Could you check a few things on this model? Use its own coordinates, in mm. A direction names the side the tool comes from. Give positions to 0.01 mm unless a question says otherwise; leave off trailing zeros. Loops run counter-clockwise (first coordinate to the right, second up) from the corner with the lowest first, then second, coordinate; pieces in that order, holes last. Notation, with made-up numbers: (-12, 65.25) - (45, 65.25) arc R9 ccw to (45, 77.25) - close; hole circle Ø2 at (-8.75, 67). An arc over 180 degrees is marked (long way). Answer in a Markdown table with one row per item. Add a question column.
Autodesk Inventor part; units mm, degrees
ref_plane "YZ Plane" through (0, 0, 0) normal (1, 0, 0) x (0, 1, 0)
ref_plane "XZ Plane" through (0, 0, 0) normal (0, 1, 0) x (-1, 0, 0)
ref_plane "XY Plane" through (0, 0, 0) normal (0, 0, 1) x (1, 0, 0)
sketch "Sketch1" plane through (0, 0, 0) normal (0, 0, 1) x (1, 0, 0)
  line L0 (0, 0) -> (114, 0)
  arc A0 (114, 0) -> (114, 18) centre (114, 9) ccw
  arc A1 (0, 21) -> (0, 0) centre (0, 10.5) ccw
  line L1 (0, 21) -> (20.7846, 18)
  line L2 (20.7846, 18) -> (114, 18)
  circle A2 centre (114, 9) radius 4.5
  dimension "d0" = 114
  dimension "d1" = 18
  dimension "d2" = 9
  dimension "d3" = 21
  dimension "d4" = 10.5
  dimension "d5" = 21
  dimension "d6" = 9
extrude "Extrusion1" add sketch "Sketch1" against normal blind 12
sketch "Sketch2" plane through (0, 0, 0) normal (0, 0, 1) x (1, 0, 0)
  line L0 (111, 0) -> (117, 0)
  line L1 (117, 0) -> (117, 6)
  line L2 (117, 6) -> (111, 6)
  line L3 (111, 6) -> (111, 0)
  point P0 (0, 0)
  dimension "d9" = 6
  dimension "d10" = 6
extrude "Extrusion2" cut sketch "Sketch2" against normal through all
sketch "Sketch3" plane through (0, 0, -12) normal (0, -1, 0) x (1, 0, 0)
  line L0 (-10.5, 12) -> (-10.5, 4)
  line L1 (-10.5, 12) -> (-10.5, 0)
  line L2 (-10.5, 4) -> (49, 4)
  line L3 (49, 4) -> (140.4404, 12)
  line L4 (140.4404, 12) -> (-10.5, 12)
  point P0 (0, 12)
  dimension "d13" = 8
  dimension "d14" = 59.5
  dimension "d15" = 175
extrude "Extrusion3" cut sketch "Sketch3" against normal through all
sketch "Sketch4" plane through (0, 0, -12) normal (0, 0, -1) x (-1, 0, 0)
  line L0 (10.5, 0) -> (-104, 0)
  line L1 (-104, 0) -> (-104, 21)
  line L2 (-104, 21) -> (10.5, 21)
  line L3 (10.5, 21) -> (10.5, 0)
  point P0 (0, 0)
  dimension "d18" = 114.5
  dimension "d19" = 21
extrude "Extrusion4" cut sketch "Sketch4" against normal through all
sketch "Sketch5" plane through (104, 0, -12) normal (-1, 0, 0) x (0, 0, 1)
  circle A0 centre (4.4, 9) radius 1.5
  point P0 (12, 0)
  dimension "d29" = 3
extrude "Extrusion5" cut sketch "Sketch5" against normal through all
fillet "Fillet1" radius 1 3 edges at (109, 18, -2.7507) (122.8704, 10.5219, -1.5372) (107.5, 0, -2.8819)
sketch "Sketch6" plane through (104, 18, -12) normal (0, 1, 0) x (1, 0, 0)
  circle A0 centre (5, -4) radius 1.5
  point P0 (-104, -12)
  dimension "d26" = 3
extrude "Extrusion6" cut sketch "Sketch6" against normal blind 5
properties part number "Hand - Digit 4"
(1) Please list where these lines run through material, in increasing order: line 1 (Y direction, x = 108.2, z = -7.6); line 2 (Y direction, x = 106.45, z = -7.6); line 3 (Y direction, x = 114, z = -9.25).
(2) On a 3-axis mill with a long thin cutter (end or side, diameter ignored), from which of +Z, -Z, +X, -X, +Y, -Y can I reach the whole of each face in a straight line? I mean faces 5 (the flat face through (109, 13, -8)), 6 (the flat face through (111, 3, -7)), 7 (the flat face through (110, 18, -6.6)). Say none if no direction works.
(3) For pin 1 Ø4.5 at (y, z) = (2, -8.5) entering from +X, with a flat end and sliding along its axis, tell me the tip position at first contact or that it passes through.
(4) We'd pull the mould along Y, two halves only. Please class faces 1 (the cylindrical face through (106.838, 7.536, -7.925)), 2 (the cylindrical face through (122.9, 10.35, -6.2)), 3 (the cylindrical face through (120.588, 7.536, -7.925)), 4 (the cylindrical face through (107.531, 0.301, -3.165)): pulls with the +Y half, pulls with the -Y half, needs draft (parallel to the pull), parting line crosses it, or undercut.
(5) I want a section at C-C on y = 9.25. State how many separate pieces and enclosed holes the cut face has, then the cut area to 3 significant figures.
(6) I want a section at A-A on z = -10.75. Please give me the cut outline in (x, y).
(7) I want a section at B-B on z = -7.6. Please give me the cut outline in (x, y), then the cut area to 3 significant figures.
Reported:
| question | item | result |
|---|---|---|
| 1 | line 1 | 0 to 7.5, 10.5 to 13 |
| 1 | line 2 | 0 to 7.5, 10.5 to 18 |
| 1 | line 3 | 13.5 to 18 |
| 2 | face 5 | +Y |
| 2 | face 6 | +Z, -Z, -Y |
| 2 | face 7 | +Z, -Z, +X, -X, +Y |
| 3 | pin 1 | x = 121.64 |
| 4 | face 1 | undercut |
| 4 | face 2 | parting line crosses it |
| 4 | face 3 | undercut |
| 4 | face 4 | pulls with the -Y half |
| 5 | separate pieces | 4 |
| 5 | enclosed holes | 0 |
| 5 | area | 66.3 mm² |
| 6 | outline | (104, 0) - (111, 0) - (111, 5.65) arc R4.5 cw (long way) to (117, 5.65) - (117, 0.51) arc R9 ccw to (114, 18) - (104, 18) - close |
| 7 | outline | (104, 0) - (111, 0) - (111, 5.65) arc R4.5 cw to (109.76, 7.5) - (104, 7.5) - close; (104, 10.5) - (109.76, 10.5) arc R4.5 cw to (118.24, 10.5) - (122.87, 10.5) arc R9 ccw to (114, 18) - (110.45, 18) - (110.45, 13) - (107.55, 13) - (107.55, 18) - (104, 18) - close; (117, 0.51) arc R9 ccw to (122.87, 7.5) - (118.24, 7.5) arc R4.5 cw to (117, 5.65) - close |
| 7 | area | 170 mm² |
